from build123d import *

# Parameters (mm, degrees)
BOSS_EXTRU_1_DEPTH      = 18.3
ESQUISSE2_W             = 14.5
ESQUISSE2_H             = 7.1
ENL_V_MAT_EXTRU_1_DEPTH = 1
ESQUISSE3_W             = 0.64
ESQUISSE3_H             = 0.64
BOSS_EXTRU_2_DEPTH      = 1
ESQUISSE4_R             = 3.5
ENL_V_MAT_EXTRU_2_DEPTH = 37.735541373


with BuildPart() as part:
    # Esquisse1 → Boss.-Extru.1 (new body)
    with BuildSketch(Plane.XY):
        with BuildLine():
            Line((-15, 13.1), (-15, -13.1))
            Line((-15, -13.1), (15, -13.1))
            Line((15, -13.1), (15, 13.1))
            ThreePointArc((15, 13.1), (0, 28.1), (-15, 13.1))
        make_face()
    extrude(amount=BOSS_EXTRU_1_DEPTH)

    # Esquisse2 → Enlèv. mat.-Extru.1 (cut)
    with BuildSketch(Plane.XZ.offset(13.1)):
        with Locations((0, 5.68)):
            Rectangle(ESQUISSE2_W, ESQUISSE2_H)
    extrude(amount=-ENL_V_MAT_EXTRU_1_DEPTH, mode=Mode.SUBTRACT)

    # Esquisse3 → Boss.-Extru.2 (add)
    with BuildSketch(Plane.XZ.offset(12.1)):
        with Locations((-5.08, 5.13)):
            Rectangle(ESQUISSE3_W, ESQUISSE3_H)
        with Locations((0, 5.13)):
            Rectangle(ESQUISSE3_W, ESQUISSE3_H)
        with Locations((2.54, 5.13)):
            Rectangle(ESQUISSE3_W, ESQUISSE3_H)
        with Locations((5.08, 5.13)):
            Rectangle(ESQUISSE3_W, ESQUISSE3_H)
        with Locations((-2.54, 5.13)):
            Rectangle(ESQUISSE3_W, ESQUISSE3_H)
    extrude(amount=BOSS_EXTRU_2_DEPTH)

    # Esquisse4 → Enlèv. mat.-Extru.2 (cut, through all)
    with BuildSketch(Plane.XY.offset(18.3)):
        with Locations((0, 13.1)):
            Circle(ESQUISSE4_R)
    extrude(amount=-ENL_V_MAT_EXTRU_2_DEPTH, mode=Mode.SUBTRACT)


solid = part.part
Source: CAD feature listing. Evaluate the final solid. Frame: model axes, mm. A direction names the side the tool comes from. Coordinates: 2 decimals unless noted, no trailing zeros. Loops run counter-clockwise (first coordinate to the right, second up) from the corner with the lowest first, then second, coordinate; pieces in that order, holes last. Notation, with made-up numbers: (69, -16.75) -> (84, -16.75) arc R10 ccw to (84, -4.75) -> close; hole circle Ø1 at (19.25, 25.25). An arc over 180 degrees is marked (long way). Answer in a Markdown table with one row per item. Add a question column.
Q1. Section B-B on x = -1.75. Return the cut outline in (y, z).
Q2. Section C-C on x = 12. Return the cut outline in (y, z), and give its area (3 significant figures).
Q3. Pull-direction query (Z, two-part tool) for faces 3 (the face through (7.25, -12.6, 5.6)), 4 (the face through (0.33, 28.096, 9.022)), 5 (the face through (-0.1, -12.6, 9.23)), 6 (the face through (0, 8, 18.3)); classes: pulls with the +Z half, pulls with the -Z half, needs draft (parallel to the pull), parting line crosses it, or undercut.
Q4. Reachability of faces 1 (the face through (-7.25, -12.6, 5.6)), 2 (the face through (-15, 0, 9)) from +Z, -Z, +X, -X, +Y, -Y: full face, straight path, thin tool, end or side. Return the list, or none.
Q5. Ray query, line 1 along Y through (x, z) = (0, 12.25); line 2 along Y through (x, z) = (0, 6.75); line 3 along X through (y, z) = (10.5, 6.5). Return the intervals inside material, ascending.
Q6. Contact query for a flat-ended pin moving along its axis: pin 1 Ø6 at (x, z) = (11.5, 12) entering from +Y. Output: stop coordinate, or through.
Q7. Section A-A on z = 3. Return the cut outline in (x, y), and give its area (3 significant figures).
Computed values:
| question | item | result |
|---|---|---|
| 1 | outline | (-13.1, 0) -> (10.07, 0) -> (10.07, 18.3) -> (-13.1, 18.3) -> (-13.1, 9.23) -> (-12.1, 9.23) -> (-12.1, 2.13) -> (-13.1, 2.13) -> close; (16.13, 0) -> (28, 0) -> (28, 18.3) -> (16.13, 18.3) -> close |
| 2 | outline | (-13.1, 0) -> (22.1, 0) -> (22.1, 18.3) -> (-13.1, 18.3) -> close |
| 2 | area | 644 mm^2 |
| 3 | face 3 | undercut |
| 3 | face 4 | needs draft |
| 3 | face 5 | undercut |
| 3 | face 6 | pulls with the +Z half |
| 4 | face 1 | -Y |
| 4 | face 2 | +Z, -Z, -X, +Y, -Y |
| 5 | line 1 | y = -13.1 to 9.6, 16.6 to 28.1 |
| 5 | line 2 | y = -12.1 to 9.6, 16.6 to 28.1 |
| 5 | line 3 | x = -15 to -2.34, 2.34 to 15 |
| 6 | pin 1 | stops at y = 25.46 |
| 7 | outline | (-15, -13.1) -> (-7.25, -13.1) -> (-7.25, -12.1) -> (7.25, -12.1) -> (7.25, -13.1) -> (15, -13.1) -> (15, 13.1) arc R15 ccw to (-15, 13.1) -> close; hole circle Ø7 at (0, 13.1) |
| 7 | area | 1,090 mm^2 |
